Verification items for the finished model (mm, model axes). Face numbers are marked on the shaded views. Round coordinates to 2 decimals unless told otherwise and drop trailing zeros. Loops run counter-clockwise (first coordinate to the right, second up) from the corner with the lowest first, then second, coordinate; pieces in that order, holes last. Notation, with made-up numbers: (40.5, 56) -> (96.5, 56) arc R18 cw to (96.5, 60) -> close; hole circle Ø9 at (46.25, -5). An arc over 180 degrees is marked (long way). Write item = value, one per line.
```python
from build123d import *

# Parameters (mm, degrees)
SKETCH1_R           = 45
BOSS_EXTRUDE1_DEPTH = 22.5
SKETCH2_R           = 45.69
BOSS_EXTRUDE2_DEPTH = 2
SKETCH3_R           = 40
SKETCH3_R_2         = 38
CUT_EXTRUDE1_DEPTH  = 32
SKETCH4_R           = 30
CUT_EXTRUDE2_DEPTH  = 82.093478159
CUT_EXTRUDE3_DEPTH  = 82.093478159


with BuildPart() as part:
    # Sketch1 → Boss-Extrude1 (new, symmetric)
    with BuildSketch(Plane(origin=(0, 0, 0), x_dir=(1, 0, 0), z_dir=(0, 1, 0))):
        with Locations(Location((0, 0, 0), (0, 0, 90))):
            Circle(SKETCH1_R)
    extrude(amount=BOSS_EXTRUDE1_DEPTH, both=True)

    # Sketch2 → Boss-Extrude2 (add)
    with BuildSketch(Plane(origin=(0, 22.5, 0), x_dir=(1, 0, 0), z_dir=(0, 1, 0))):
        with Locations(Location((0, 0, 0), (0, 0, 270))):
            Circle(SKETCH2_R)
    boss_extrude2 = extrude(amount=BOSS_EXTRUDE2_DEPTH)

    # Mirror1: Boss-Extrude2 across plane
    add(boss_extrude2.mirror(Plane.ZX))

    # Sketch3 → Cut-Extrude1 (cut)
    with BuildSketch(Plane(origin=(0, 0, 0), x_dir=(1, 0, 0), z_dir=(0, 1, 0))):
        with Locations(Location((0, 0, 0), (0, 0, 270))):
            Circle(SKETCH3_R)
        with Locations(Location((0, 0, 0), (0, 0, 270))):
            Circle(SKETCH3_R_2, mode=Mode.SUBTRACT)
    extrude(amount=-CUT_EXTRUDE1_DEPTH, mode=Mode.SUBTRACT)

    # Sketch4 → Cut-Extrude2 (cut, through all)
    with BuildSketch(Plane.XZ.offset(24.5)):
        with Locations(Location((0, 0, 0), (0, 0, 270))):
            Circle(SKETCH4_R)
    extrude(amount=-CUT_EXTRUDE2_DEPTH, mode=Mode.SUBTRACT)

    # Sketch6 → Cut-Extrude3 (cut, through all)
    with BuildSketch(Plane.XZ.offset(24.5)):
        with BuildLine():
            Line((-9, 28.618176043), (-9, 33.20180718))
            ThreePointArc((-9, 33.20180718), (0, 34.4), (9, 33.20180718))
            Line((9, 33.20180718), (9, 28.618176043))
            ThreePointArc((9, 28.618176043), (0, 30), (-9, 28.618176043))
        make_face()
    extrude(amount=-CUT_EXTRUDE3_DEPTH, mode=Mode.SUBTRACT)


solid = part.part
```
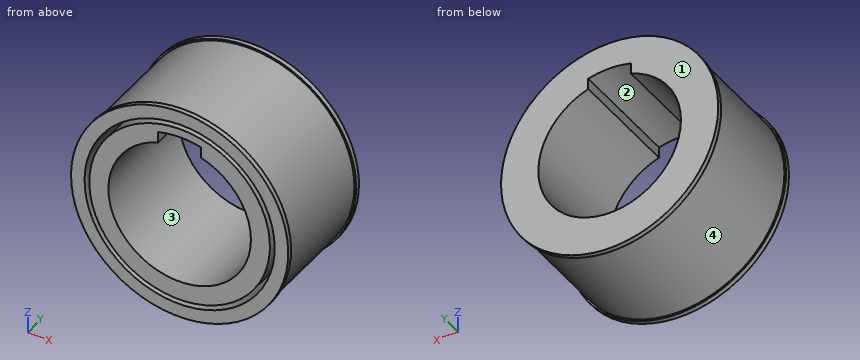
(1) Sectioned sample at D-D, the plane y = 7.5. Record the cut outline in (x, z).
Filled sheet:
outline = circle Ø90 at (0, 0); hole (-9, 28.62) arc R30 ccw (long way) to (9, 28.62) -> (9, 33.2) arc R34.4 ccw to (-9, 33.2) -> close
(2) Material ranges on probe 1 along X at (y, z) = (-15, 0); probe 2 along Z at (x, y) = (32, -8); probe 3 along X at (y, z) = (-8, -34), recorded low to high. Write a range as from..to.
Filled sheet:
probe_1 = -45..-40, -38..-30, 30..38, 40..45
probe_2 = -31.64..-24, -20.49..20.49, 24..31.64
probe_3 = -29.48..-21.07, -16.97..16.97, 21.07..29.48
(3) Sectioned sample at B-B, the plane x = 0. Record the cut outline in (y, z), and give its area (3 significant figures).
Filled sheet:
outline = (-24.5, -45.69) -> (-22.5, -45.69) -> (-22.5, -45) -> (22.5, -45) -> (22.5, -45.69) -> (24.5, -45.69) -> (24.5, -30) -> (-24.5, -30) -> (-24.5, -38) -> (0, -38) -> (0, -40) -> (-24.5, -40) -> close; (-24.5, 34.4) -> (24.5, 34.4) -> (24.5, 45.69) -> (22.5, 45.69) -> (22.5, 45) -> (-22.5, 45) -> (-22.5, 45.69) -> (-24.5, 45.69) -> (-24.5, 40) -> (0, 40) -> (0, 38) -> (-24.5, 38) -> close
area = 1,160 mm2
(4) Go/stop test with flat-tipped pins: pin 1 Ø1.5 at (y, z) = (18, -19) entering from -X; pin 2 Ø4 at (y, z) = (15.5, -25.5) entering from -X; pin 3 Ø1 at (x, y) = (-5.5, 7) entering from -Z. Record where each tip stops, or that it passes through.
Filled sheet:
pin_1 = -41.13
pin_2 = -38.38
pin_3 = -44.72
(5) Draft check along X on the marked faces 1, 2, 3 and 4. Enter one of: released by +X, released by -X, zero draft, split by the parting line, or undercut.
Filled sheet:
face_1 = zero draft
face_2 = undercut
face_3 = undercut
face_4 = split by the parting line
(6) Sectioned sample at C-C, the plane y = -5.5. Record the cut outline in (x, z).
Filled sheet:
outline = circle Ø90 at (0, 0); circle Ø76 at (0, 0); hole circle Ø80 at (0, 0); hole (-9, 28.62) arc R30 ccw (long way) to (9, 28.62) -> (9, 33.2) arc R34.4 ccw to (-9, 33.2) -> close
(7) Sectioned sample at A-A, the plane z = 0. Record the cut outline in (x, y), and give its area (3 significant figures).
Filled sheet:
outline = (-45.69, -24.5) -> (-40, -24.5) -> (-40, 0) -> (-38, 0) -> (-38, -24.5) -> (-30, -24.5) -> (-30, 24.5) -> (-45.69, 24.5) -> (-45.69, 22.5) -> (-45, 22.5) -> (-45, -22.5) -> (-45.69, -22.5) -> close; (30, -24.5) -> (38, -24.5) -> (38, 0) -> (40, 0) -> (40, -24.5) -> (45.69, -24.5) -> (45.69, -22.5) -> (45, -22.5) -> (45, 22.5) -> (45.69, 22.5) -> (45.69, 24.5) -> (30, 24.5) -> close
area = 1,380 mm2
